Geometry: final body of the model. Coordinates: model frame, mm. A direction names the side the tool comes from. Round coordinates to 2 decimals unless told otherwise and drop trailing zeros. Loops run counter-clockwise (first coordinate to the right, second up) from the corner with the lowest first, then second, coordinate; pieces in that order, holes last. Notation, with made-up numbers: (7.25, 53) -> (46.25, 53) arc R14 cw to (46.25, 76) -> close; hole circle Ø8 at (-15.5, -16). An arc over 180 degrees is marked (long way). Answer in a Markdown table with one row per item.
Autodesk Inventor part; units mm, degrees
ref_plane "YZ Plane" through (0, 0, 0) normal (1, 0, 0) x (0, 1, 0)
ref_plane "XZ Plane" through (0, 0, 0) normal (0, 1, 0) x (-1, 0, 0)
ref_plane "XY Plane" through (0, 0, 0) normal (0, 0, 1) x (1, 0, 0)
sketch "Sketch1" plane through (0, 0, 0) normal (0, 1, 0) x (-1, 0, 0)
  line L0 (0, 0) -> (88.9, 0)
  line L1 (88.9, 0) -> (88.9, -88.9)
  line L2 (88.9, -88.9) -> (0, -88.9)
  line L3 (0, -88.9) -> (0, 0)
  dimension "d0" = 88.9
  dimension "d1" = 88.9
extrude "Extrusion1" add sketch "Sketch1" along normal blind 6.35
shell "Shell1" thickness 5.969 removed faces 1 at (-29.6333, 6.35, -29.6333)
sketch "Sketch2" plane through (0, 6.35, 0) normal (0, 1, 0) x (1, 0, 0)
  circle A0 centre (-44.45, 3.1115) radius 1.5875
  line L0 (-88.9, 88.9) -> (-88.9, 0)
  line L1 (-5.969, 5.969) -> (-82.931, 5.969)
  circle A1 centre (-86.0425, 44.45) radius 1.5875
  line L2 (-88.9, 0) -> (0, 0)
  circle A2 centre (-2.8575, 44.45) radius 1.5875
  line L3 (0, 0) -> (0, 88.9)
  circle A3 centre (-46.0375, 85.7885) radius 1.5875
  line L4 (-82.931, 82.931) -> (-5.969, 82.931)
  dimension "d8" = 3.175
  dimension "d10" = 2.8575
  dimension "d11" = 3.175
  dimension "d12" = 2.8575
  dimension "d13" = 44.45
  dimension "d14" = 3.175
  dimension "d15" = 2.8575
  dimension "d16" = 3.175
  dimension "d17" = 2.8575
extrude "Extrusion2" cut sketch "Sketch2" against normal blind 3.175
properties part number "bottom plate"
Item 1: First-contact query: P1, Ø23, axis at x = -43, z = -28.5, coming from the +Y side; P2, Ø1.6, axis at x = -3, z = -44, coming from the +Y side (3 decimals). Flat tips, straight axial feed; report the tip coordinate or a pass-through.
Ans:
| item | result |
|---|---|
| P1 | y = 5.97 |
| P2 | y = 3.175 |
Item 2: Section query C-C, the plane z = -44.45. Output: boundary loops of the cut face in (x, y) (3 decimals), and give its area (3 significant figures).
Ans:
| item | result |
|---|---|
| outline | (-88.9, 0) -> (0, 0) -> (0, 6.35) -> (-1.27, 6.35) -> (-1.27, 3.175) -> (-4.445, 3.175) -> (-4.445, 6.35) -> (-5.969, 6.35) -> (-5.969, 5.969) -> (-82.931, 5.969) -> (-82.931, 6.35) -> (-84.455, 6.35) -> (-84.455, 3.175) -> (-87.63, 3.175) -> (-87.63, 6.35) -> (-88.9, 6.35) -> close |
| area | 515 mm2 |
Item 3: Ray query, L1, parallel to X at y = 4.55, z = -44.45 (3 decimals); L2, parallel to Y at x = -36, z = -45. Return the intervals inside material, ascending.
Ans:
| item | result |
|---|---|
| L1 | -88.9 to -87.63, -84.455 to -4.445, -1.27 to 0 |
| L2 | 0 to 5.97 |
Item 4: Mould query, pull axis X, two halves, no side actions, for faces 1 (the flat face through (-44, 3, 0)), 2 (the flat face through (-86, 3.175, -44)), 3 (the cylindrical face through (-86.39, 4.78, -42.9)), 4 (the flat face through (-88.9, 3, -44)). Classes: released by +X, released by -X, zero draft, split by the parting line, or undercut.
Ans:
| item | result |
|---|---|
| face 1 | zero draft |
| face 2 | undercut |
| face 3 | undercut |
| face 4 | released by -X |
Item 5: Section query A-A, the plane z = -24.5. Output: boundary loops of the cut face in (x, y).
Ans:
| item | result |
|---|---|
| outline | (-88.9, 0) -> (0, 0) -> (0, 6.35) -> (-5.97, 6.35) -> (-5.97, 5.97) -> (-82.93, 5.97) -> (-82.93, 6.35) -> (-88.9, 6.35) -> close |
Item 6: Section query B-B, the plane x = -24. Output: boundary loops of the cut face in (y, z), and give its area (3 significant figures).
Ans:
| item | result |
|---|---|
| outline | (0, -88.9) -> (6.35, -88.9) -> (6.35, -82.93) -> (5.97, -82.93) -> (5.97, -5.97) -> (6.35, -5.97) -> (6.35, 0) -> (0, 0) -> close |
| area | 535 mm2 |
Item 7: Set-up query: faces 5 (the flat face through (-46, 3.175, -86)), 6 (the flat face through (-44, 0, -44)). Return all of +Z, -Z, +X, -X, +Y, -Y with unobstructed straight access to the full face (end or side cutting, diameter ignored); none if empty.
Ans:
| item | result |
|---|---|
| face 5 | +Y |
| face 6 | +Z, -Z, +X, -X, -Y |
